from build123d import *

# Parameters (mm, degrees)
SKETCH1_R           = 8.509
SKETCH1_R_2         = 4.445
BOSS_EXTRUDE1_DEPTH = 15.24
FILLET1_R           = 0.762
SKETCH2_R           = 0.635
CUT_EXTRUDE1_DEPTH  = 1.27


with BuildPart() as part:
    # Sketch1 → Boss-Extrude1 (new body)
    with BuildSketch(Plane.XY):
        Circle(SKETCH1_R)
        Circle(SKETCH1_R_2, mode=Mode.SUBTRACT)
    extrude(amount=BOSS_EXTRUDE1_DEPTH)

    # Fillet1
    fillet1_edges = [part.edges().sort_by_distance(p)[0] for p in [
        (-8.509, 0, 0),
        (-8.509, 0, 15.24),
    ]]
    fillet(fillet1_edges, radius=FILLET1_R)

    # Sketch2 → Cut-Extrude1 (cut)
    with BuildSketch(Plane.XY.offset(15.24)):
        with Locations((0, 6.35)):
            Circle(SKETCH2_R)
        with Locations((2.755161743, 5.721152311)):
            Circle(SKETCH2_R)
        with Locations((4.964629914, 3.959160242)):
            Circle(SKETCH2_R)
        with Locations((6.190792242, 1.413007931)):
            Circle(SKETCH2_R)
        with Locations((6.190792242, -1.413007931)):
            Circle(SKETCH2_R)
        with Locations((4.964629914, -3.959160242)):
            Circle(SKETCH2_R)
        with Locations((2.755161743, -5.721152311)):
            Circle(SKETCH2_R)
        with Locations((0, -6.35)):
            Circle(SKETCH2_R)
        with Locations((-2.755161743, -5.721152311)):
            Circle(SKETCH2_R)
        with Locations((-4.964629914, -3.959160242)):
            Circle(SKETCH2_R)
        with Locations((-6.190792242, -1.413007931)):
            Circle(SKETCH2_R)
        with Locations((-6.190792242, 1.413007931)):
            Circle(SKETCH2_R)
        with Locations((-4.964629914, 3.959160242)):
            Circle(SKETCH2_R)
        with Locations((-2.755161743, 5.721152311)):
            Circle(SKETCH2_R)
    extrude(amount=-CUT_EXTRUDE1_DEPTH, mode=Mode.SUBTRACT)


solid = part.part
For this review, take the finished solid that the model builds, in its own axes (mm). Give positions to 0.01 mm unless a question says otherwise; leave off trailing zeros. Order: outer loops, then holes, each group sorted by start corner. A loop starts at its lowest first (then second) coordinate and runs counter-clockwise, first axis right, second up. Notation, with made-up numbers: M 7.25,-34 L 18.25,-34 A23 cw 18.25,-8 Z; hole C 61.25,77.5 d3. An arc over 180 degrees is marked long. Answer in a Markdown table with one row per item. Add a question column.
(1) Consider section B-B on y = 0. State the section outline as (x, z) points (3 decimals).
(2) Wall thickness on probe 1 along X at (y, z) = (-0.5, 7.5); probe 2 along Y at (x, z) = (1.5, 5.5): over which ranges is each line inside the solid? List them lowest first. Write a range as [from, to].
(3) Mouldability with a two-part tool opening along Y and no side actions: class faces 1 (the face through (2.62, -6.34, 14.61)), 2 (the face through (-1.108, 8.437, 7.524)) as +Y half, -Y half, draft (parallel to the pull), parting line (faces both ways), or undercut.
(4) Consider section A-A on x = 0. State the section outline as (y, z) points (3 decimals), and give its area (3 significant figures).
(5) Consider section C-C on z = 7.25. State the section outline as (x, y) points (3 decimals).
(6) For pin 1 (0.6 mm diameter, centred on x = 5, y = 4, fed in from +Z); pin 2 (1 mm diameter, centred on y = 1, z = 11, fed in from +X); pin 3 (5 mm diameter, centred on y = -3, z = 3, fed in from -X), all flat-tipped, find the tip position at first contact; note any pin that passes through.
Evaluation:
| question | item | result |
|---|---|---|
| 1 | outline | M -8.509,0.762 A0.762 ccw -7.747,0 L -4.445,0 L -4.445,15.24 L -7.747,15.24 A0.762 ccw -8.509,14.478 Z; M 4.445,0 L 7.747,0 A0.762 ccw 8.509,0.762 L 8.509,14.478 A0.762 ccw 7.747,15.24 L 4.445,15.24 Z |
| 2 | probe 1 | x = [-8.49, -4.42], [4.42, 8.49] |
| 2 | probe 2 | y = [-8.38, -4.18], [4.18, 8.38] |
| 3 | face 1 | undercut |
| 3 | face 2 | parting line |
| 4 | outline | M -8.509,0.762 A0.762 ccw -7.747,0 L -4.445,0 L -4.445,15.24 L -5.715,15.24 L -5.715,13.97 L -6.985,13.97 L -6.985,15.24 L -7.747,15.24 A0.762 ccw -8.509,14.478 Z; M 4.445,0 L 7.747,0 A0.762 ccw 8.509,0.762 L 8.509,14.478 A0.762 ccw 7.747,15.24 L 6.985,15.24 L 6.985,13.97 L 5.715,13.97 L 5.715,15.24 L 4.445,15.24 Z |
| 4 | area | 120 mm^2 |
| 5 | outline | C 0,0 d17.018; hole C 0,0 d8.89 |
| 6 | pin 1 | stops at z = 13.97 |
| 6 | pin 2 | stops at x = 8.49 |
| 6 | pin 3 | stops at x = -8.49 |
